Read the model definition and answer for the solid it produces. Units are mm, in the model's axes. Coordinates: 2 decimals unless noted, no trailing zeros. Write each loop counter-clockwise with the first axis right and the second up, starting at its lowest first coordinate (ties: lowest second). Pieces come first, ordered by that corner, then holes.
(1) Section B-B on z = 258 is taken. Write down the section's boundary in (x, y), then the cut area to 3 significant figures.
(2) Given pin 1 (15 mm diameter, centred on x = 56, z = 21, fed in from -Y); pin 2 (5 mm diameter, centred on x = -12, y = -27, fed in from -Z); pin 3 (9 mm diameter, centred on x = -12, z = 18.5, fed in from +Y); pin 4 (8 mm diameter, centred on x = -90, y = -105, fed in from +Z), each flat-ended and moving along its own axis, determine where each tip first touches the part or whether it passes through.
(3) Find the intervals of material crossed by probe 1 along Y at (x, z) = (-90, -1); probe 2 along Y at (x, z) = (90, 15); probe 3 along Y at (x, z) = (-6.5, 519), in increasing order.
(4) Section A-A on x = -64 is taken. Write down the section's boundary in (y, z), then the cut area to 3 significant figures.
from build123d import *

# Parameters (mm, degrees)
SKETCH1_W           = 60
SKETCH1_H           = 50
BOSS_EXTRUDE1_DEPTH = 30
SKETCH2_W           = 30
SKETCH2_H           = 30
BOSS_EXTRUDE2_DEPTH = 700
SKETCH3_R           = 6
BOSS_EXTRUDE3_DEPTH = 7
CUT_EXTRUDE1_REACH  = 732
SKETCH4_R           = 6.523816089


with BuildPart() as part:
    # Sketch1 → Boss-Extrude1 (new body)
    with BuildSketch(Plane.XY):
        Polygon((-105, 125), (-75, 125), (-75, 55), (75, 55), (75, 125), (105, 125), (105, -125), (75, -125), (75, -55), (-75, -55), (-75, -125), (-105, -125), align=None)
        with Locations((-45, 0)):
            Rectangle(SKETCH1_W, SKETCH1_H, mode=Mode.SUBTRACT)
        with Locations((45, 0)):
            Rectangle(SKETCH1_W, SKETCH1_H, mode=Mode.SUBTRACT)
    extrude(amount=BOSS_EXTRUDE1_DEPTH)

    # Sketch2 → Boss-Extrude2 (add)
    with BuildSketch(Plane.XY.offset(30)):
        Rectangle(SKETCH2_W, SKETCH2_H)
    extrude(amount=BOSS_EXTRUDE2_DEPTH)

    # Sketch3 → Boss-Extrude3 (add)
    with BuildSketch(Plane(origin=(0, 0, 0), x_dir=(-1, 0, 0), z_dir=(0, 0, -1))):
        Polygon((81.339745962, 110), (90, 115), (98.660254038, 110), (98.660254038, 100), (90, 95), (81.339745962, 100), align=None)
        with Locations((90, 105)):
            Circle(SKETCH3_R, mode=Mode.SUBTRACT)
        Polygon((-90, 115), (-98.660254038, 110), (-98.660254038, 100), (-90, 95), (-81.339745962, 100), (-81.339745962, 110), align=None)
        with Locations((-90, 105)):
            Circle(SKETCH3_R, mode=Mode.SUBTRACT)
        Polygon((81.339745962, -100), (81.339745962, -110), (90, -115), (98.660254038, -110), (98.660254038, -100), (90, -95), align=None)
        with Locations((90, -105)):
            Circle(SKETCH3_R, mode=Mode.SUBTRACT)
        Polygon((-81.339745962, -110), (-90, -115), (-98.660254038, -110), (-98.660254038, -100), (-90, -95), (-81.339745962, -100), align=None)
        with Locations((-90, -105)):
            Circle(SKETCH3_R, mode=Mode.SUBTRACT)
    extrude(amount=BOSS_EXTRUDE3_DEPTH)

    # Sketch4 → Cut-Extrude1 (cut, up to next)
    with BuildSketch(Plane(origin=(0, 0, 0), x_dir=(-1, 0, 0), z_dir=(0, 0, -1)), mode=Mode.PRIVATE) as cut_extrude1_sk1:
        with Locations((-90, 105)):
            Circle(SKETCH4_R)
    cut_extrude1_tool1 = extrude(cut_extrude1_sk1.sketch, amount=-CUT_EXTRUDE1_REACH, mode=Mode.PRIVATE) & part.part
    add(cut_extrude1_tool1.solids().sort_by_distance((90, 105, 0))[0], mode=Mode.SUBTRACT)
    # Sketch4 → Cut-Extrude1 (cut, up to next)
    with BuildSketch(Plane(origin=(0, 0, 0), x_dir=(-1, 0, 0), z_dir=(0, 0, -1)), mode=Mode.PRIVATE) as cut_extrude1_sk2:
        with Locations((90, 105)):
            Circle(SKETCH4_R)
    cut_extrude1_tool2 = extrude(cut_extrude1_sk2.sketch, amount=-CUT_EXTRUDE1_REACH, mode=Mode.PRIVATE) & part.part
    add(cut_extrude1_tool2.solids().sort_by_distance((-90, 105, 0))[0], mode=Mode.SUBTRACT)
    # Sketch4 → Cut-Extrude1 (cut, up to next)
    with BuildSketch(Plane(origin=(0, 0, 0), x_dir=(-1, 0, 0), z_dir=(0, 0, -1)), mode=Mode.PRIVATE) as cut_extrude1_sk3:
        with Locations((90, -105)):
            Circle(SKETCH4_R)
    cut_extrude1_tool3 = extrude(cut_extrude1_sk3.sketch, amount=-CUT_EXTRUDE1_REACH, mode=Mode.PRIVATE) & part.part
    add(cut_extrude1_tool3.solids().sort_by_distance((-90, -105, 0))[0], mode=Mode.SUBTRACT)
    # Sketch4 → Cut-Extrude1 (cut, up to next)
    with BuildSketch(Plane(origin=(0, 0, 0), x_dir=(-1, 0, 0), z_dir=(0, 0, -1)), mode=Mode.PRIVATE) as cut_extrude1_sk4:
        with Locations((-90, -105)):
            Circle(SKETCH4_R)
    cut_extrude1_tool4 = extrude(cut_extrude1_sk4.sketch, amount=-CUT_EXTRUDE1_REACH, mode=Mode.PRIVATE) & part.part
    add(cut_extrude1_tool4.solids().sort_by_distance((90, -105, 0))[0], mode=Mode.SUBTRACT)


solid = part.part
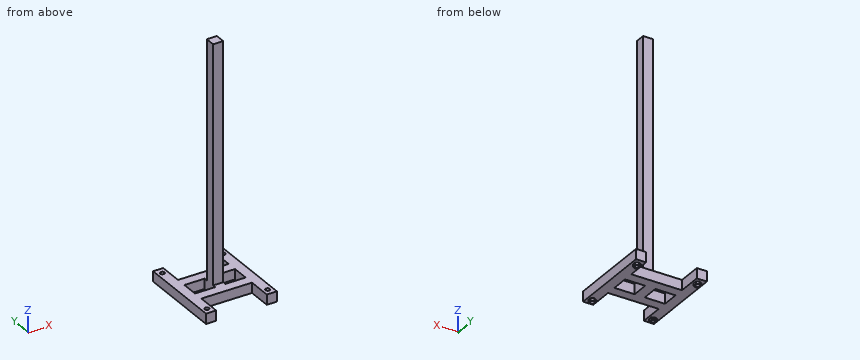
Response:
1. outline: (-15, -15) - (15, -15) - (15, 15) - (-15, 15) - close
1. area: 900 mm2
2. pin 1: stops at y = -55
2. pin 2: stops at z = 0
2. pin 3: stops at y = 55
2. pin 4: passes through
3. probe 1: y = -115 to -111, -99 to -95, 95 to 99, 111 to 115
3. probe 2: y = -125 to -111.52, -98.48 to 98.48, 111.52 to 125
3. probe 3: y = -15 to 15
4. outline: (-55, 0) - (-25, 0) - (-25, 30) - (-55, 30) - close; (25, 0) - (55, 0) - (55, 30) - (25, 30) - close
4. area: 1,800 mm2
